from build123d import *

# Parameters (mm, degrees)
SKETCH1_W                                           = 115
SKETCH1_H                                           = 45
BOSS_EXTRUDE1_DEPTH                                 = 5
CUT_EXTRUDE1_REACH                                  = 119.287
SKETCH2_R                                           = 9.8171
CSK_FOR_M2_COUNTERSUNK_FLAT_HEAD_SCREW1_D           = 2.4
CSK_FOR_M2_COUNTERSUNK_FLAT_HEAD_SCREW1_CSINK_D     = 5.4
CSK_FOR_M2_COUNTERSUNK_FLAT_HEAD_SCREW1_CSINK_ANGLE = 90
SKETCH13_W                                          = 52
SKETCH13_H                                          = 45
BOSS_EXTRUDE4_DEPTH                                 = 6
CHAMFER2_SIZE                                       = 6
M3_TAPPED_HOLE1_D                                   = 2.5
CHAMFER1_SIZE                                       = 3
SKETCH14_W                                          = 10
SKETCH14_H                                          = 30
BOSS_EXTRUDE5_DEPTH                                 = 5
FILLET1_R                                           = 2
CSK_FOR_M2_COUNTERSUNK_FLAT_HEAD_SCREW2_D           = 2.4
CSK_FOR_M2_COUNTERSUNK_FLAT_HEAD_SCREW2_DEPTH       = 5
CSK_FOR_M2_COUNTERSUNK_FLAT_HEAD_SCREW2_CSINK_D     = 5.4
CSK_FOR_M2_COUNTERSUNK_FLAT_HEAD_SCREW2_CSINK_ANGLE = 90
CSK_FOR_M2_COUNTERSUNK_FLAT_HEAD_SCREW2_TIP         = 0.721032743
SKETCH17_W                                          = 3
SKETCH17_H                                          = 3
BOSS_EXTRUDE6_DEPTH                                 = 6


with BuildPart() as part:
    # Sketch1 → Boss-Extrude1 (new body)
    with BuildSketch(Plane(origin=(0, 0, 0), x_dir=(1, 0, 0), z_dir=(0, 1, 0))):
        with Locations((57.5, 0)):
            Rectangle(SKETCH1_W, SKETCH1_H)
    extrude(amount=BOSS_EXTRUDE1_DEPTH)

    # Sketch2 → Cut-Extrude1 (cut, up to next)
    with BuildSketch(Plane(origin=(0, 5, 0), x_dir=(1, 0, 0), z_dir=(0, 1, 0)), mode=Mode.PRIVATE) as cut_extrude1_sk1:
        with Locations(Location((22.5, 0, 0), (0, 0, 270))):
            Circle(SKETCH2_R)
    cut_extrude1_tool1 = extrude(cut_extrude1_sk1.sketch, amount=-CUT_EXTRUDE1_REACH, mode=Mode.PRIVATE) & part.part
    add(cut_extrude1_tool1.solids().sort_by_distance((22.5, 5, 0))[0], mode=Mode.SUBTRACT)

    # CSK for M2 Countersunk Flat Head Screw1 (through all)
    with Locations(Plane(origin=(0, 5, 0), x_dir=(1, 0, 0), z_dir=(0, 1, 0))):
        with Locations((4, -18.5), (41, -18.5), (41, 5), (4, 5)):
            CounterSinkHole(CSK_FOR_M2_COUNTERSUNK_FLAT_HEAD_SCREW1_D / 2, CSK_FOR_M2_COUNTERSUNK_FLAT_HEAD_SCREW1_CSINK_D / 2, counter_sink_angle=CSK_FOR_M2_COUNTERSUNK_FLAT_HEAD_SCREW1_CSINK_ANGLE)

    # Sketch13 → Boss-Extrude4 (add)
    with BuildSketch(Plane(origin=(0, 5, 0), x_dir=(1, 0, 0), z_dir=(0, 1, 0))):
        with Locations((89, 0)):
            Rectangle(SKETCH13_W, SKETCH13_H)
    extrude(amount=BOSS_EXTRUDE4_DEPTH)

    # Chamfer2
    chamfer2_edges = [part.edges().sort_by_distance(p)[0] for p in [
        (63, 11, 0),
    ]]
    chamfer(chamfer2_edges, length=CHAMFER2_SIZE - 0.0001)  # a hair under: the kernel refuses the full size

    # M3 Tapped Hole1 (through all)
    with Locations(Plane(origin=(0, 11, 0), x_dir=(1, 0, 0), z_dir=(0, 1, 0))):
        with Locations((83, 16), (111, 16), (83, -16), (111, -16)):
            Hole(M3_TAPPED_HOLE1_D / 2)

    # Chamfer1
    chamfer1_edges = [part.edges().sort_by_distance(p)[0] for p in [
        (115, 5.5, -22.5),
        (115, 5.5, 22.5),
    ]]
    chamfer(chamfer1_edges, length=CHAMFER1_SIZE)

    # Sketch14 → Boss-Extrude5 (add)
    with BuildSketch(Plane(origin=(0, 0, 0), x_dir=(1, 0, 0), z_dir=(0, 1, 0))):
        with Locations((-5, 0)):
            Rectangle(SKETCH14_W, SKETCH14_H)
    extrude(amount=BOSS_EXTRUDE5_DEPTH)

    # Fillet1
    fillet1_edges = [part.edges().sort_by_distance(p)[0] for p in [
        (0, 2.5, -15),
        (0, 2.5, 15),
    ]]
    fillet(fillet1_edges, radius=FILLET1_R)

    # CSK for M2 Countersunk Flat Head Screw2
    with Locations(Plane(origin=(0, 0, 0), x_dir=(-1, 0, 0), z_dir=(0, -1, 0))):
        with Locations((-1.5, 0), (6, -10), (6, 10)):
            CounterSinkHole(CSK_FOR_M2_COUNTERSUNK_FLAT_HEAD_SCREW2_D / 2, CSK_FOR_M2_COUNTERSUNK_FLAT_HEAD_SCREW2_CSINK_D / 2, depth=CSK_FOR_M2_COUNTERSUNK_FLAT_HEAD_SCREW2_DEPTH, counter_sink_angle=CSK_FOR_M2_COUNTERSUNK_FLAT_HEAD_SCREW2_CSINK_ANGLE)
            with Locations((0, 0, -(CSK_FOR_M2_COUNTERSUNK_FLAT_HEAD_SCREW2_DEPTH + CSK_FOR_M2_COUNTERSUNK_FLAT_HEAD_SCREW2_TIP / 2))):  # 118° drill point
                Cone(0, CSK_FOR_M2_COUNTERSUNK_FLAT_HEAD_SCREW2_D / 2, CSK_FOR_M2_COUNTERSUNK_FLAT_HEAD_SCREW2_TIP, mode=Mode.SUBTRACT)

    # Sketch17 → Boss-Extrude6 (add)
    with BuildSketch(Plane(origin=(0, 5, 0), x_dir=(1, 0, 0), z_dir=(0, 1, 0))):
        with Locations((-6, 0)):
            Rectangle(SKETCH17_W, SKETCH17_H)
    extrude(amount=BOSS_EXTRUDE6_DEPTH)


solid = part.part
CAD build for the part. Positions are in the model's coordinates, mm. A direction names the side the tool comes from. Coordinates: 2 decimals unless noted, no trailing zeros. Order: outer loops, then holes, each group sorted by start corner. A loop starts at its lowest first (then second) coordinate and runs counter-clockwise, first axis right, second up. Notation, with made-up numbers: (37.25, -2.5) -> (59.25, -2.5) arc R27 cw to (59.25, 27.5) -> close; hole circle Ø7 at (-1.75, 85). An arc over 180 degrees is marked (long way). Answer in a Markdown table with one row per item.
1) Mould opens along X. For faces 1 (the face through (-6.26, 3.27, -8.83)), 2 (the face through (-6, 8, -1.5)), 3 (the face through (0, 2, -20)), 4 (the face through (-4.5, 8, 0)) say: pulls with the +X half, pulls with the -X half, needs draft (parallel to the pull), parting line crosses it, or undercut.
Check values:
| item | result |
|---|---|
| face 1 | undercut |
| face 2 | needs draft |
| face 3 | pulls with the -X half |
| face 4 | undercut |
2) Drill centre lines: line 1 (Z direction, x = 83, y = 8.5); line 2 (X direction, y = 0.7, z = 18.5); line 3 (Z direction, x = 41, y = 1.75). Where is each one in solid material? Low to high.
Check values:
| item | result |
|---|---|
| line 1 | -22.5 to -17.25, -14.75 to 14.75, 17.25 to 22.5 |
| line 2 | 0 to 2.8, 5.2 to 39.8, 42.2 to 115 |
| line 3 | -22.5 to -6.2, -3.8 to 17.3, 19.7 to 22.5 |
3) Band-saw the part on B-B (z = 0). Give the number of separate pieces and of enclosed holes in the cut face, and give its area (3 significant figures).
Check values:
| item | result |
|---|---|
| separate pieces | 3 |
| enclosed holes | 0 |
| area | 825 mm2 |
4) Band-saw the part on C-C (x = 83). List the corners of the cut face in (y, z).
Check values:
| item | result |
|---|---|
| outline | (0, -22.5) -> (11, -22.5) -> (11, -17.25) -> (0, -17.25) -> close; (0, -14.75) -> (11, -14.75) -> (11, 14.75) -> (0, 14.75) -> close; (0, 17.25) -> (11, 17.25) -> (11, 22.5) -> (0, 22.5) -> close |
5) Flat gauge pins, fed straight in: P1, Ø22.5, axis at x = 33.5, z = 5.5, coming from the +Y side; P2, Ø5, axis at y = 8, z = 15, coming from the -X side; P3, Ø2.5, axis at x = -4, y = 3, coming from the -Z side. Where does each tip first touch, or does it go through?
Check values:
| item | result |
|---|---|
| P1 | y = 5 |
| P2 | x = 63.5 |
| P3 | z = -15 |
6) Band-saw the part on A-A (y = 8.75). List the corners of the cut face in (x, z), and give its area (3 significant figures).
Check values:
| item | result |
|---|---|
| outline | (-7.5, -1.5) -> (-4.5, -1.5) -> (-4.5, 1.5) -> (-7.5, 1.5) -> close; (66.75, -22.5) -> (112, -22.5) -> (115, -19.5) -> (115, 19.5) -> (112, 22.5) -> (66.75, 22.5) -> close; hole circle Ø2.5 at (83, -16); hole circle Ø2.5 at (83, 16); hole circle Ø2.5 at (111, -16); hole circle Ø2.5 at (111, 16) |
| area | 2,150 mm2 |
7) Which spindle directions (+Z, -Z, +X, -X, +Y, -Y) get a long thin tool onto all of the face, cutting with end or side? Do faces 5 (the face through (-6, 8, 1.5)), 6 (the face through (92, 11, 0)). Say none if no direction does.
Check values:
| item | result |
|---|---|
| face 5 | +Z, -X, +Y |
| face 6 | +Z, -Z, +X, -X, +Y |
